```python
from build123d import *

# Parameters (mm, degrees)
BAR_DEPTH           = 150
CUT_EXTRUDE4_DEPTH  = 5
CUT_EXTRUDE3_REACH  = 19.238
SKETCH6_W           = 48.933333333
SKETCH6_H           = 12.2
SKETCH6_W_2         = 48.933333334
BOSS_EXTRUDE2_DEPTH = 0.8


with BuildPart() as part:
    # Sketch1 → Bar (new body)
    with BuildSketch(Plane(origin=(0, 0, 0), x_dir=(0, 0, -1), z_dir=(1, 0, 0))):
        with BuildLine():
            Line((7.238093672, -6.9), (7.238093672, 6.9))
            ThreePointArc((7.238093672, 6.9), (-10, 0), (7.238093672, -6.9))
        make_face()
        Polygon((1, 6.573205081), (-1.005255888, 7.730940108), (-4.9, 5.482308546), (-4.9, -5.482308546), (-1.005255888, -7.730940108), (1, -6.573205081), align=None, mode=Mode.SUBTRACT)
    extrude(amount=-BAR_DEPTH)

    # Sketch10 → Cut-Extrude4 (cut)
    with BuildSketch(Plane.ZY.offset(150)):
        with BuildLine():
            Line((-6.238093672, -6.487386788), (-6.238093672, 6.487386788))
            ThreePointArc((-6.238093672, 6.487386788), (9, 0), (-6.238093672, -6.487386788))
        make_face()
    extrude(amount=-CUT_EXTRUDE4_DEPTH, mode=Mode.SUBTRACT)

    # Sketch6 → Cut-Extrude3 (cut, up to next)
    with BuildSketch(Plane(origin=(0, 0, -7.238093672), x_dir=(1, 0, 0), z_dir=(0, 0, -1)), mode=Mode.PRIVATE) as cut_extrude3_sk1:
        with Locations((-25.266666667, 0)):
            Rectangle(SKETCH6_W, SKETCH6_H)
    cut_extrude3_tool1 = extrude(cut_extrude3_sk1.sketch, amount=-CUT_EXTRUDE3_REACH, mode=Mode.PRIVATE) & part.part
    add(cut_extrude3_tool1.solids().sort_by_distance((-25.266667, 0, -7.238094))[0], mode=Mode.SUBTRACT)
    # Sketch6 → Cut-Extrude3 (cut, up to next)
    with BuildSketch(Plane(origin=(0, 0, -7.238093672), x_dir=(1, 0, 0), z_dir=(0, 0, -1)), mode=Mode.PRIVATE) as cut_extrude3_sk2:
        with Locations((-75, 0)):
            Rectangle(SKETCH6_W_2, SKETCH6_H)
    cut_extrude3_tool2 = extrude(cut_extrude3_sk2.sketch, amount=-CUT_EXTRUDE3_REACH, mode=Mode.PRIVATE) & part.part
    add(cut_extrude3_tool2.solids().sort_by_distance((-75, 0, -7.238094))[0], mode=Mode.SUBTRACT)
    # Sketch6 → Cut-Extrude3 (cut, up to next)
    with BuildSketch(Plane(origin=(0, 0, -7.238093672), x_dir=(1, 0, 0), z_dir=(0, 0, -1)), mode=Mode.PRIVATE) as cut_extrude3_sk3:
        with Locations((-124.733333334, 0)):
            Rectangle(SKETCH6_W, SKETCH6_H)
    cut_extrude3_tool3 = extrude(cut_extrude3_sk3.sketch, amount=-CUT_EXTRUDE3_REACH, mode=Mode.PRIVATE) & part.part
    add(cut_extrude3_tool3.solids().sort_by_distance((-124.733333, 0, -7.238094))[0], mode=Mode.SUBTRACT)

    # Sketch11 → Boss-Extrude2 (add)
    with BuildSketch(Plane(origin=(0, 0, 0), x_dir=(0, 0, -1), z_dir=(1, 0, 0))):
        with BuildLine():
            Line((7.238093672, -6.9), (7.238093672, 6.9))
            ThreePointArc((7.238093672, 6.9), (-10, 0), (7.238093672, -6.9))
        make_face()
    extrude(amount=-BOSS_EXTRUDE2_DEPTH)


solid = part.part
```
Geometry check sheet. Reference: the model listing, model coordinates, mm. A direction names the side the tool comes from. Give positions to 0.01 mm unless a question says otherwise; leave off trailing zeros. Order: outer loops, then holes, each group sorted by start corner. A loop starts at its lowest first (then second) coordinate and runs counter-clockwise, first axis right, second up. Notation, with made-up numbers: (16.5, 9) - (58.5, 9) arc R19 ccw to (58.5, 31) - close; hole circle Ø6 at (79.5, 32). An arc over 180 degrees is marked (long way). Answer in a Markdown table with one row per item. Add a question column.
Q1. Mould release check, pull along Y, two halves, no side actions. Record for faces 4 (the flat face through (-50.533, 0, -4)), 5 (the flat face through (-75, -6.1, -4)), 6 (the flat face through (0, 0, 2)): pulls with the +Y half, pulls with the -Y half, needs draft (parallel to the pull), parting line crosses it, or undercut.
Q2. Tool access check on faces 1 (the flat face through (-74.6, -6.7, -7.238)), 2 (the flat face through (-49.733, 0, -4)), 3 (the flat face through (-149.4, 0, -6.238)). Record the directions out of +Z, -Z, +X, -X, +Y, -Y that give a thin tool (end or side, any length) a straight path to the whole face; none if there is none.
Q3. Gauge pin test, flat ends, axial feed: pin 1 (3 mm diameter, centred on x = -118.5, z = -2.5, fed in from +Y); pin 2 (7 mm diameter, centred on x = -113.5, z = -5, fed in from -Y); pin 3 (1 mm diameter, centred on x = -94.5, y = -5.5, fed in from -Z); pin 4 (8 mm diameter, centred on x = -16, z = -1, fed in from +Y). Record the tip position at first contact, or that the pin passes through.
Q4. Cross-section at A-A, the plane y = 0. Enter the section's corners in (x, z).
Q5. Cross-section at B-B, the plane x = -78.5. Enter the section's corners in (y, z).
Q6. Cross-section at C-C, the plane z = 6.5. Enter the section's corners in (x, y).
Q7. Material ranges on probe 1 along X at (y, z) = (-3.5, -4.75); probe 2 along Y at (x, z) = (-147.8, 0); probe 3 along X at (y, z) = (-7, -2), recorded low to high. Write a range as from..to.
Q8. Cross-section at D-D, the plane z = -2.5. Enter the section's corners in (x, y), then the cut area to 3 significant figures.
Check values:
| question | item | result |
|---|---|---|
| 1 | face 4 | undercut |
| 1 | face 5 | undercut |
| 1 | face 6 | needs draft |
| 2 | face 1 | -Z, +X, -X, +Y, -Y |
| 2 | face 2 | -Z |
| 2 | face 3 | -X |
| 3 | pin 1 | stops at y = 9.95 |
| 3 | pin 2 | stops at y = -9.89 |
| 3 | pin 3 | stops at z = 4 |
| 3 | pin 4 | stops at y = 10 |
| 4 | outline | (-150, -7.24) - (-149.2, -7.24) - (-149.2, -6.24) - (-150, -6.24) - close; (-150, 9) - (-145, 9) - (-145, 4.9) - (-0.8, 4.9) - (-0.8, -7.24) - (0, -7.24) - (0, 10) - (-150, 10) - close; (-100.27, -7.24) - (-99.47, -7.24) - (-99.47, -1) - (-100.27, -1) - close; (-50.53, -7.24) - (-49.73, -7.24) - (-49.73, -1) - (-50.53, -1) - close |
| 5 | outline | (-7.73, 1.01) - (-5.48, 4.9) - (5.48, 4.9) - (7.73, 1.01) - (6.57, -1) - (6.1, -1) - (6.1, -7.24) - (6.9, -7.24) arc R10 ccw (long way) to (-6.9, -7.24) - (-6.1, -7.24) - (-6.1, -1) - (-6.57, -1) - close |
| 6 | outline | (-150, -7.6) - (0, -7.6) - (0, 7.6) - (-150, 7.6) - (-150, 6.22) - (-145, 6.22) - (-145, -6.22) - (-150, -6.22) - close |
| 7 | probe 1 | x = -100.27..-99.47, -50.53..-49.73, -0.8..0 |
| 7 | probe 2 | y = -10..-9, 9..10 |
| 7 | probe 3 | x = -145..0 |
| 8 | outline | (-150, -9.68) - (0, -9.68) - (0, 9.68) - (-150, 9.68) - (-150, 8.65) - (-145, 8.65) - (-145, 6.1) - (-100.27, 6.1) - (-100.27, -6.1) - (-145, -6.1) - (-145, -8.65) - (-150, -8.65) - close; hole (-99.47, -6.1) - (-50.53, -6.1) - (-50.53, 6.1) - (-99.47, 6.1) - close; hole (-49.73, -6.1) - (-0.8, -6.1) - (-0.8, 6.1) - (-49.73, 6.1) - close |
| 8 | area | 1,080 mm^2 |
